```python
from build123d import *

# Parameters (mm, degrees)
PAD_DEPTH          = 8
POCKET_DEPTH       = 6
SKETCH002_R        = 2.5
SKETCH002_W        = 10
SKETCH002_H        = 5.5
POCKET001_DEPTH    = 2
SKETCH012_W        = 3
SKETCH012_H        = 6.5
PAD004_DEPTH       = 0.4
SKETCH003_W        = 12
SKETCH003_H        = 1.5
SKETCH003_W_2      = 1.5
SKETCH003_H_2      = 10
SKETCH003_H_3      = 12
POCKET002_DEPTH    = 5
CHAMFER_SIZE       = 1
SKETCH013_W        = 15.5
SKETCH013_H        = 1.5
POCKET003_DEPTH    = 3.5
CHAMFER002_SIZE    = 1
SKETCH014_W        = 10
SKETCH014_H        = 2
SKETCH014_W_2      = 3
SKETCH014_W_3      = 2
SKETCH014_H_2      = 5
PAD005_DEPTH       = 3
SKETCH015_W        = 7.5
SKETCH015_H        = 7.5
PAD006_DEPTH       = 5
SKETCH016_R        = 1.45
POCKET004_DEPTH    = 7
CHAMFER003_SIZE    = 1.5
CHAMFER004_1_SIZE2 = 2.9
CHAMFER004_1_SIZE  = 1.9
CHAMFER004_2_SIZE2 = 2.9
CHAMFER004_2_SIZE  = 1.9
CHAMFER004_3_SIZE2 = 2.9
CHAMFER004_3_SIZE  = 1.9
CHAMFER005_SIZE2   = 1.9
CHAMFER005_SIZE    = 2.9
CHAMFER007_SIZE    = 0.4
CHAMFER008_SIZE    = 1


with BuildPart() as part:
    # Sketch → Pad (new body)
    with BuildSketch(Plane.XY):
        with BuildLine():
            Line((-40.5, -27), (40.5, -27))
            ThreePointArc((40.5, -27), (43.681981, -25.681981), (45, -22.5))
            Line((45, -22.5), (45, 22.5))
            ThreePointArc((45, 22.5), (43.681981, 25.681981), (40.5, 27))
            Line((40.5, 27), (-40.5, 27))
            ThreePointArc((-40.5, 27), (-43.681981, 25.681981), (-45, 22.5))
            Line((-45, 22.5), (-45, -22.5))
            ThreePointArc((-45, -22.5), (-43.681981, -25.681981), (-40.5, -27))
        make_face()
    extrude(amount=PAD_DEPTH)

    # Sketch001 (on Face10 of Pad) → Pocket (cut)
    with BuildSketch(Plane.XY.offset(8)):
        with BuildLine():
            Line((-39, -25.5), (39, -25.5))
            ThreePointArc((39, -25.5), (42.181981, -24.181981), (43.5, -21))
            Line((43.5, -21), (43.5, 21))
            ThreePointArc((43.5, 21), (42.181981, 24.181981), (39, 25.5))
            Line((39, 25.5), (-39, 25.5))
            ThreePointArc((-39, 25.5), (-42.181981, 24.181981), (-43.5, 21))
            Line((-43.5, 21), (-43.5, -21))
            ThreePointArc((-43.5, -21), (-42.181981, -24.181981), (-39, -25.5))
        make_face()
    extrude(amount=-POCKET_DEPTH, mode=Mode.SUBTRACT)

    # Sketch002 (on Face4 of Pocket) → Pocket001 (cut)
    with BuildSketch(Plane(origin=(0, 0, 0), x_dir=(1, 0, 0), z_dir=(0, 0, -1))):
        with Locations((-12.5, 13)):
            Circle(SKETCH002_R)
        Polygon((-16, -23.5), (-32, -23.5), (-32, -17), (-16, -17), (-16, -16), (-33, -16), (-33, -24.5), (-16, -24.5), align=None)
        with Locations((15.25, -22.75)):
            Rectangle(SKETCH002_W, SKETCH002_H)
    extrude(amount=-POCKET001_DEPTH, mode=Mode.SUBTRACT)

    # Sketch012 (on Face30 of Pocket001) → Pad004 (join)
    with BuildSketch(Plane.XY.offset(2)):
        with Locations((-30.5, 20.25)):
            Rectangle(SKETCH012_W, SKETCH012_H)
    extrude(amount=PAD004_DEPTH)

    # Sketch003 (on Face5 of Pocket001) → Pocket002 (cut)
    with BuildSketch(Plane.XY.offset(8)):
        with Locations((-11.75, -26.25)):
            Rectangle(SKETCH003_W, SKETCH003_H)
        with Locations((44.25, -9.5)):
            Rectangle(SKETCH003_W_2, SKETCH003_H_2)
        with Locations((-27.75, -26.25)):
            Rectangle(SKETCH003_W, SKETCH003_H)
        with Locations((44.25, 9)):
            Rectangle(SKETCH003_W_2, SKETCH003_H_3)
    extrude(amount=-POCKET002_DEPTH, mode=Mode.SUBTRACT)

    # Chamfer
    chamfer_edges = [part.edges().sort_by_distance(p)[0] for p in [
        (44.25, -4.5, 3),
        (-17.75, -26.25, 3),
        (-5.75, -26.25, 3),
        (44.25, -14.5, 3),
        (-33.75, -26.25, 3),
        (44.25, 15, 3),
        (44.25, 3, 3),
        (-21.75, -26.25, 3),
    ]]
    chamfer(chamfer_edges, length=CHAMFER_SIZE)

    # Sketch013 (on Face4 of Chamfer) → Pocket003 (cut)
    with BuildSketch(Plane.XY.offset(8)):
        with Locations((5.5, -26.25)):
            Rectangle(SKETCH013_W, SKETCH013_H)
    extrude(amount=-POCKET003_DEPTH, mode=Mode.SUBTRACT)

    # Chamfer002
    chamfer002_edges = [part.edges().sort_by_distance(p)[0] for p in [
        (-2.25, -26.25, 4.5),
        (13.25, -26.25, 4.5),
    ]]
    chamfer(chamfer002_edges, length=CHAMFER002_SIZE)

    # Sketch014 (on Face51 of Chamfer002) → Pad005 (join)
    with BuildSketch(Plane.XY.offset(2)):
        with Locations((19, -24.5)):
            Rectangle(SKETCH014_W, SKETCH014_H)
        with Locations((-4, -24.5)):
            Rectangle(SKETCH014_W_2, SKETCH014_H)
        with Locations((-19.75, -24.5)):
            Rectangle(SKETCH014_W_2, SKETCH014_H)
        with Locations((42.5, -1)):
            Rectangle(SKETCH014_W_3, SKETCH014_H_2)
    extrude(amount=PAD005_DEPTH)

    # Sketch015 (on Face51 of Pad005) → Pad006 (join)
    with BuildSketch(Plane.XY.offset(2)):
        with Locations((39.75, 21.75)):
            Rectangle(SKETCH015_W, SKETCH015_H)
        with Locations((-39.75, -21.75)):
            Rectangle(SKETCH015_W, SKETCH015_H)
        with Locations((-39.75, 21.75)):
            Rectangle(SKETCH015_W, SKETCH015_H)
        with Locations((39.75, -21.75)):
            Rectangle(SKETCH015_W, SKETCH015_H)
    extrude(amount=PAD006_DEPTH)

    # Sketch016 (on Face83 of Pad006) → Pocket004 (cut)
    with BuildSketch(Plane.XY.offset(7)):
        with Locations((-39, 21)):
            Circle(SKETCH016_R)
        with Locations((39, 21)):
            Circle(SKETCH016_R)
        with Locations((39, -21)):
            Circle(SKETCH016_R)
        with Locations((-39, -21)):
            Circle(SKETCH016_R)
    extrude(amount=-POCKET004_DEPTH, mode=Mode.SUBTRACT)

    # Chamfer003
    chamfer003_edges = [part.edges().sort_by_distance(p)[0] for p in [
        (-36, 18, 4.5),
        (36, 18, 4.5),
        (36, -18, 4.5),
        (-36, -18, 4.5),
    ]]
    chamfer(chamfer003_edges, length=CHAMFER003_SIZE)

    # Chamfer004 1
    chamfer004_1_edges = [part.edges().sort_by_distance(p)[0] for p in [
        (19, -23.5, 5),
    ]]
    chamfer004_1_side = part.faces().sort_by_distance((19, -24.5, 5))[0]
    chamfer(chamfer004_1_edges, length=CHAMFER004_1_SIZE, length2=CHAMFER004_1_SIZE2, reference=chamfer004_1_side)

    # Chamfer004 2
    chamfer004_2_edges = [part.edges().sort_by_distance(p)[0] for p in [
        (-4, -23.5, 5),
    ]]
    chamfer004_2_side = part.faces().sort_by_distance((-4, -24.5, 5))[0]
    chamfer(chamfer004_2_edges, length=CHAMFER004_2_SIZE, length2=CHAMFER004_2_SIZE2, reference=chamfer004_2_side)

    # Chamfer004 3
    chamfer004_3_edges = [part.edges().sort_by_distance(p)[0] for p in [
        (-19.75, -23.5, 5),
    ]]
    chamfer004_3_side = part.faces().sort_by_distance((-19.75, -24.5, 5))[0]
    chamfer(chamfer004_3_edges, length=CHAMFER004_3_SIZE, length2=CHAMFER004_3_SIZE2, reference=chamfer004_3_side)

    # Chamfer005
    chamfer005_edges = [part.edges().sort_by_distance(p)[0] for p in [
        (41.5, -1, 5),
    ]]
    chamfer005_side = part.faces().sort_by_distance((41.5, -1, 3.5))[0]
    chamfer(chamfer005_edges, length=CHAMFER005_SIZE, length2=CHAMFER005_SIZE2, reference=chamfer005_side)

    # Chamfer007
    chamfer007_edges = [part.edges().sort_by_distance(p)[0] for p in [
        (-40.45, 21, 7),
        (37.55, -21, 7),
        (-40.45, -21, 7),
        (37.55, 21, 7),
        (-36, -22.5, 7),
        (-36.75, -18.75, 7),
        (-40.5, -18, 7),
        (-40.5, 18, 7),
        (-36.75, 18.75, 7),
        (-36, 22.5, 7),
        (36, -22.5, 7),
        (36.75, -18.75, 7),
        (40.5, -18, 7),
        (40.5, 18, 7),
        (36.75, 18.75, 7),
        (36, 22.5, 7),
        (37.55, -21, 0),
        (37.55, 21, 0),
        (15.25, 20, 0),
        (20.25, 22.75, 0),
        (15.25, 25.5, 0),
        (10.25, 22.75, 0),
        (-24, 17, 0),
        (-32, 20.25, 0),
        (-24, 23.5, 0),
        (-16, 24, 0),
        (-24.5, 24.5, 0),
        (-33, 20.25, 0),
        (-24.5, 16, 0),
        (-16, 16.5, 0),
        (-40.45, 21, 0),
        (-40.45, -21, 0),
        (-15, -13, 0),
    ]]
    chamfer(chamfer007_edges, length=CHAMFER007_SIZE)

    # Chamfer008
    chamfer008_edges = [part.edges().sort_by_distance(p)[0] for p in [
        (0, -27, 0),
    ]]
    chamfer(chamfer008_edges, length=CHAMFER008_SIZE)


solid = part.part
```
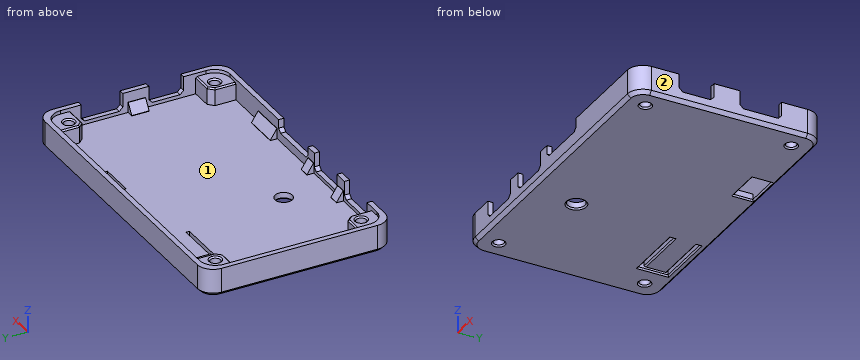
Check sheet for the modelled part. Datum: model origin and axes. Units: mm. Face numbers are marked on the shaded views. A direction names the side the tool comes from. Give positions to 0.01 mm unless a question says otherwise; leave off trailing zeros. Loops run counter-clockwise (first coordinate to the right, second up) from the corner with the lowest first, then second, coordinate; pieces in that order, holes last. Notation, with made-up numbers: (50, 16) - (60, 16) arc R17 ccw to (60, 46) - close; hole circle Ø9 at (-3, -23). An arc over 180 degrees is marked (long way). One line per question, with ' | ' between items. Start each with the question number.
1. Cross-section at A-A, the plane x = 16.5. Enter the section's corners in (y, z), plus the area to 3 significant figures.
2. Material ranges on line 1 along Y through (x, z) = (39, 5); line 2 along X through (y, z) = (19.5, 1.75); line 3 along Y through (x, z) = (-12.5, 1.35), recorded low to high. Write a range as [from, to].
3. Cross-section at D-D, the plane x = 31. Enter the section's corners in (y, z).
4. Gauge pin test, flat ends, axial feed: pin 1 Ø1.6 at (x, y) = (44, -8.5) entering from +Z; pin 2 Ø1.6 at (y, z) = (-26.5, 6) entering from -X; pin 3 Ø1.2 at (y, z) = (-26.5, 5) entering from -X; pin 4 Ø8 at (x, y) = (38.5, -23.5) entering from +Z. Record the tip position at first contact, or that the pin passes through.
5. Cross-section at B-B, the plane x = -30. Enter the section's corners in (y, z).
6. Cross-section at C-C, the plane y = 0. Enter the section's corners in (x, z).
7. Set-up check for the marked faces 1 and 2: record each of +Z, -Z, +X, -X, +Y, -Y from which the full face is reachable in a straight line by a thin tool's end or side.
Check result:
1) outline: (-27, 1) - (-26, 0) - (19.6, 0) - (20, 0.4) - (20, 2) - (-23.5, 2) - (-23.5, 2.1) - (-25.4, 5) - (-25.5, 5) - (-25.5, 8) - (-27, 8) - close; (25.5, 0.4) - (25.9, 0) - (26, 0) - (27, 1) - (27, 8) - (25.5, 8) - close | area: 117 mm2
2) line 1: y = [-27, -22.45], [-19.55, -18], [18, 19.55], [22.45, 27] | line 2: x = [-45, -33], [-32, 45] | line 3: y = [-27, -15.5], [-10.5, 27]
3) outline: (-27, 1) - (-26, 0) - (26, 0) - (27, 1) - (27, 8) - (25.5, 8) - (25.5, 2) - (-25.5, 2) - (-25.5, 8) - (-27, 8) - close
4) pin 1: stops at z = 3 | pin 2: stops at x = -43.66 | pin 3: stops at x = -43.45 | pin 4: stops at z = 8
5) outline: (-27, 1) - (-26, 0) - (15.6, 0) - (16, 0.4) - (16, 2) - (-25.5, 2) - (-25.5, 3) - (-27, 3) - close; (17, 0.4) - (17.4, 0) - (23.1, 0) - (23.5, 0.4) - (23.5, 2.4) - (17, 2.4) - close; (24.5, 0.4) - (24.9, 0) - (26, 0) - (27, 1) - (27, 8) - (25.5, 8) - (25.5, 2) - (24.5, 2) - close
6) outline: (-45, 1) - (-44, 0) - (44, 0) - (45, 1) - (45, 8) - (43.5, 8) - (43.5, 5) - (43.4, 5) - (41.5, 2.1) - (41.5, 2) - (-43.5, 2) - (-43.5, 8) - (-45, 8) - close
7) face 1: +Z | face 2: +Z, -Z, +X, +Y, -Y
